Build history of the part. All positions in model axes, mm. Face numbers are marked on the shaded views. A direction names the side the tool comes from. Coordinates: 2 decimals unless noted, no trailing zeros. Write each loop counter-clockwise with the first axis right and the second up, starting at its lowest first coordinate (ties: lowest second). Pieces come first, ordered by that corner, then holes.
```python
from build123d import *

# Parameters (mm, degrees)
PAD001_DEPTH = 1
CHAMFER_SIZE = 0.5
PAD_DEPTH    = 20
POCKET_DEPTH = 19


with BuildPart() as chamfer_body:
    # Sketch003 → Pad001 (new body)
    with BuildSketch(Plane.XY.offset(11)):
        with BuildLine():
            ThreePointArc((0, 5.9), (-5.9, 0), (0, -5.9))
            Line((0, -5.9), (11.8, -5.9))
            ThreePointArc((11.8, -5.9), (17.7, 0), (11.8, 5.9))
            Line((0, 5.9), (11.8, 5.9))
        make_face()
        with BuildLine():
            ThreePointArc((0, 4.9), (-4.9, 0), (0, -4.9))
            Line((0, -4.9), (11.8, -4.9))
            ThreePointArc((11.8, -4.9), (16.7, 0), (11.8, 4.9))
            Line((0, 4.9), (11.8, 4.9))
        make_face(mode=Mode.SUBTRACT)
    extrude(amount=PAD001_DEPTH)

    # Chamfer
    chamfer_edges = [chamfer_body.edges().sort_by_distance(p)[0] for p in [
        (5.9, -5.9, 12),
        (-5.9, 0, 12),
        (17.7, 0, 12),
        (5.9, 5.9, 12),
    ]]
    chamfer(chamfer_edges, length=CHAMFER_SIZE)


with BuildPart() as fusion:
    # Sketch → Pad (new body)
    with BuildSketch(Plane.XY):
        with BuildLine():
            ThreePointArc((0, 4.9), (-4.9, 0), (0, -4.9))
            Line((0, -4.9), (11.8, -4.9))
            ThreePointArc((11.8, -4.9), (16.7, 0), (11.8, 4.9))
            Line((0, 4.9), (11.8, 4.9))
        make_face()
    extrude(amount=PAD_DEPTH)

    # Sketch001 → Pocket (cut)
    with BuildSketch(Plane(origin=(0, 0, 0), x_dir=(1, 0, 0), z_dir=(0, 0, -1))):
        with BuildLine():
            ThreePointArc((0, 3.65), (-3.65, 0), (0, -3.65))
            Line((0, -3.65), (11.8, -3.65))
            ThreePointArc((11.8, -3.65), (15.45, 0), (11.8, 3.65))
            Line((0, 3.65), (11.8, 3.65))
        make_face()
    extrude(amount=-POCKET_DEPTH, mode=Mode.SUBTRACT)

    # Fusion: union Chamfer body
    add(chamfer_body.part)


solid = fusion.part
```
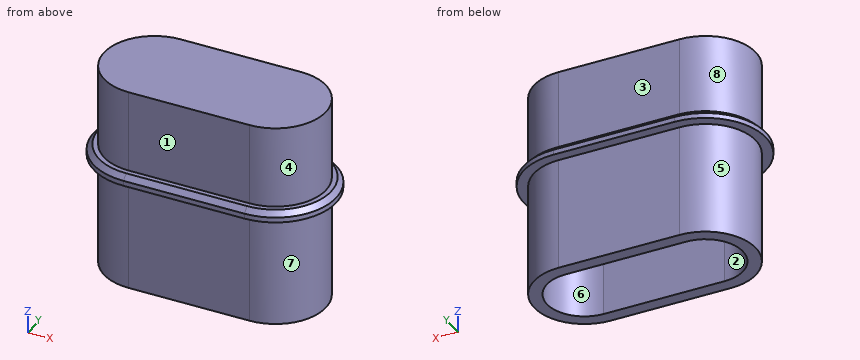
1. Saw through at B-B on x = 4.75. List the corners of the cut face in (y, z), plus the area to 4 significant figures.
Computed values:
outline: (-5.9, 11) - (-4.9, 11) - (-4.9, 0) - (-3.65, 0) - (-3.65, 19) - (3.65, 19) - (3.65, 0) - (4.9, 0) - (4.9, 11) - (5.9, 11) - (5.9, 11.5) - (5.4, 12) - (4.9, 12) - (4.9, 20) - (-4.9, 20) - (-4.9, 12) - (-5.4, 12) - (-5.9, 11.5) - close
area: 59.05 mm2
2. Flat gauge pins, fed straight in: pin 1 (1.5 mm diameter, centred on x = 3.5, z = 17, fed in from +Y); pin 2 (1.5 mm diameter, centred on x = -1.5, z = 8, fed in from +Y); pin 3 (3.5 mm diameter, centred on x = 7, y = 0.5, fed in from -Z). Where does each tip first touch, or does it go through?
Computed values:
pin 1: stops at y = 4.9
pin 2: stops at y = 4.84
pin 3: stops at z = 19
3. Mould opens along Y. For the marked faces 1, 2, 3 and 4 say: +Y half, -Y half, draft (parallel to the pull), parting line (faces both ways), or undercut.
Computed values:
face 1: -Y half
face 2: undercut
face 3: +Y half
face 4: parting line
4. 3-axis set-ups, long thin cutter, end or side, ignore diameter. For the marked faces 5, 6, 7 and 8: which of +Z, -Z, +X, -X, +Y, -Y reach the whole face in a straight line?
Computed values:
face 5: -Z, -X
face 6: -Z
face 7: -Z, +X
face 8: +Z, -X
5. Saw through at A-A on y = 0. List the corners of the cut face in (x, z).
Computed values:
outline: (-5.9, 11) - (-4.9, 11) - (-4.9, 0) - (-3.65, 0) - (-3.65, 19) - (15.45, 19) - (15.45, 0) - (16.7, 0) - (16.7, 11) - (17.7, 11) - (17.7, 11.5) - (17.2, 12) - (16.7, 12) - (16.7, 20) - (-4.9, 20) - (-4.9, 12) - (-5.4, 12) - (-5.9, 11.5) - close
6. Probe line 1 along Y through (x, z) = (4, 9); line 2 along Z through (x, y) = (4, 5.25); line 3 along X through (y, z) = (-1.25, 10.5). List the from-to ranges inside material, lowest first.
Computed values:
line 1: y = -4.9 to -3.65, 3.65 to 4.9
line 2: z = 11 to 12
line 3: x = -4.74 to -3.43, 15.23 to 16.54
